from build123d import *

# Parameters (mm, degrees)
SKETCH1_W           = 35
SKETCH1_H           = 20
SKETCH1_R           = 1.5
BOSS_EXTRUDE1_DEPTH = 1.53
SKETCH2_R           = 10
BOSS_EXTRUDE2_DEPTH = 15
SKETCH3_R           = 9
SKETCH3_R_2         = 4
CUT_EXTRUDE1_DEPTH  = 0.5
SKETCH4_W           = 2.5
SKETCH4_H           = 10
BOSS_EXTRUDE3_DEPTH = 2.5


with BuildPart() as part:
    # Sketch1 → Boss-Extrude1 (new body)
    with BuildSketch(Plane(origin=(0, 0, 0), x_dir=(1, 0, 0), z_dir=(0, 1, 0))):
        with Locations((17.5, 10)):
            Rectangle(SKETCH1_W, SKETCH1_H)
        with Locations((32.75, 17.75)):
            Circle(SKETCH1_R, mode=Mode.SUBTRACT)
        with Locations((32.75, 2.25)):
            Circle(SKETCH1_R, mode=Mode.SUBTRACT)
    extrude(amount=BOSS_EXTRUDE1_DEPTH)

    # Sketch2 → Boss-Extrude2 (add)
    with BuildSketch(Plane(origin=(0, 1.53, 0), x_dir=(1, 0, 0), z_dir=(0, 1, 0))):
        with Locations((10, 10)):
            Circle(SKETCH2_R)
    extrude(amount=BOSS_EXTRUDE2_DEPTH)

    # Sketch3 → Cut-Extrude1 (cut)
    with BuildSketch(Plane(origin=(0, 16.53, 0), x_dir=(1, 0, 0), z_dir=(0, 1, 0))):
        with Locations((10, 10)):
            Circle(SKETCH3_R)
        with Locations((10, 10)):
            Circle(SKETCH3_R_2, mode=Mode.SUBTRACT)
    extrude(amount=-CUT_EXTRUDE1_DEPTH, mode=Mode.SUBTRACT)

    # Sketch4 → Boss-Extrude3 (add)
    with BuildSketch(Plane(origin=(0, 1.53, 0), x_dir=(1, 0, 0), z_dir=(0, 1, 0))):
        with Locations((32.75, 10)):
            Rectangle(SKETCH4_W, SKETCH4_H)
    extrude(amount=BOSS_EXTRUDE3_DEPTH)


solid = part.part
Source: CAD feature listing. Evaluate the final solid. Frame: model axes, mm. A direction names the side the tool comes from. Round coordinates to 2 decimals unless told otherwise and drop trailing zeros. Loops run counter-clockwise (first coordinate to the right, second up) from the corner with the lowest first, then second, coordinate; pieces in that order, holes last. Notation, with made-up numbers: (61.25, 64.5) -> (77.25, 64.5) arc R27 ccw to (77.25, 83.5) -> close; hole circle Ø6 at (62, -20). An arc over 180 degrees is marked (long way). Answer as a JSON object with one key per item and string values. Group by question number.
Q1. Mould query, pull axis Z, two halves, no side actions, for faces 4 (the flat face through (17, 1, 0)), 5 (the cylindrical face through (31.25, 0.75, -2.32)), 6 (the flat face through (25, 1.53, -10)), 7 (the cylindrical face through (31.64, 0.75, -18.76)). Classes: pulls with the +Z half, pulls with the -Z half, needs draft (parallel to the pull), parting line crosses it, or undercut.
Q2. Section query A-A (y = 2.75). Output: boundary loops of the cut face in (x, z), plus the area to 3 significant figures.
Q3. Access query for faces 1 (the flat face through (33, 4.03, -10)), 2 (the cylindrical face through (6.004, 16.284, -10.176)), 3 (the flat face through (33, 3, -5)). Directions: +Z, -Z, +X, -X, +Y, -Y. A direction counts if a zero-diameter tool reaches every point of the face in a straight line with its end or side. Return the directions, or none.
Q4. Ray query, line 1 (Z direction, x = 32.75, y = 1.2); line 2 (Z direction, x = 10, y = 16.25); line 3 (X direction, y = 0.95, z = -17.75). Return the intervals inside material, ascending. Write a range as from..to.
Q5. Contact query for flat-ended pins moving along their axis: P1, Ø6, axis at y = 14, z = -3, coming from the -X side; P2, Ø2, axis at x = 32.5, z = -12, coming from the +Y side; P3, Ø1.8, axis at x = 32.75, z = -2.25, coming from the -Y side; P4, Ø8, axis at x = 20.5, y = 10.5, coming from the -Z side. Output: stop coordinate, or through.
Q6. Section query B-B (x = 32.75). Output: boundary loops of the cut face in (y, z), plus the area to 3 significant figures.
Q7. Section query D-D (x = 4.5). Output: boundary loops of the cut face in (y, z), plus the area to 3 significant figures.
Q8. Section query C-C (z = -2.25). Output: boundary loops of the cut face in (x, y), plus the area to 3 significant figures.
Completed:
{
 "1": {"face 4": "pulls with the +Z half", "face 5": "undercut", "face 6": "needs draft", "face 7": "undercut"},
 "2": {"outline": "circle Ø20 at (10, -10); (31.5, -15) -> (34, -15) -> (34, -5) -> (31.5, -5) -> close", "area": "339 mm²"},
 "3": {"face 1": "+Z, -Z, +X, +Y", "face 2": "+Y", "face 3": "+Z, +X, +Y"},
 "4": {"line 1": "-20..-19.25, -16.25..-3.75, -0.75..0", "line 2": "-20..-19, -14..-6, -1..0", "line 3": "0..31.25, 34.25..35"},
 "5": {"P1": "x = 0.83", "P2": "y = 4.03", "P3": "through", "P4": "z = -17.6"},
 "6": {"outline": "(0, -20) -> (1.53, -20) -> (1.53, -19.25) -> (0, -19.25) -> close; (0, -16.25) -> (1.53, -16.25) -> (1.53, -15) -> (4.03, -15) -> (4.03, -5) -> (1.53, -5) -> (1.53, -3.75) -> (0, -3.75) -> close; (0, -0.75) -> (1.53, -0.75) -> (1.53, 0) -> (0, 0) -> close", "area": "46.4 mm²"},
 "7": {"outline": "(0, -20) -> (1.53, -20) -> (1.53, -18.35) -> (16.53, -18.35) -> (16.53, -17.12) -> (16.03, -17.12) -> (16.03, -2.88) -> (16.53, -2.88) -> (16.53, -1.65) -> (1.53, -1.65) -> (1.53, 0) -> (0, 0) -> close", "area": "274 mm²"},
 "8": {"outline": "(0, 0) -> (31.25, 0) -> (31.25, 1.53) -> (16.32, 1.53) -> (16.32, 16.53) -> (14.58, 16.53) -> (14.58, 16.03) -> (5.42, 16.03) -> (5.42, 16.53) -> (3.68, 16.53) -> (3.68, 1.53) -> (0, 1.53) -> close; (34.25, 0) -> (35, 0) -> (35, 1.53) -> (34.25, 1.53) -> close", "area": "234 mm²"}
}
